```python
from build123d import *

# Parameters (mm, degrees)
BODY_SKETCH_W       = 31.8
BODY_SKETCH_H       = 20.9
BODY_DEPTH          = 9.9
NUT_X_SKETCH_W      = 16.85
NUT_X_SKETCH_H      = 9.45
NUT_X_SKETCH_2_W    = 16.85
NUT_X_SKETCH_2_H    = 9.45
SOCKET_X_SKETCH_W   = 17.8
SOCKET_X_SKETCH_H   = 4.7625
SOCKET_X_SKETCH_2_W = 17.8
SOCKET_X_SKETCH_2_H = 4.7625


with BuildPart() as part:
    # Body Sketch → Body (new, symmetric)
    with BuildSketch(Plane.XY):
        with Locations((0, 0.75)):
            Rectangle(BODY_SKETCH_W, BODY_SKETCH_H)
    extrude(amount=BODY_DEPTH, both=True)

    # Nut _X Sketch → Nut _X (revolve)
    with BuildSketch(Plane.XY, mode=Mode.PRIVATE) as nut_x_sk:
        with Locations((24.325, 4.725)):
            Rectangle(NUT_X_SKETCH_W, NUT_X_SKETCH_H)
    revolve(nut_x_sk.sketch.rotate(Axis((-1000, 0, 0), (1, 0, 0)), 90), axis=Axis((-1000, 0, 0), (1, 0, 0)))

    # Nut -X Sketch 2 → Nut -X 2 (revolve)
    with BuildSketch(Plane.XY, mode=Mode.PRIVATE) as nut_x_2_sk:
        with Locations((-24.325, 4.725)):
            Rectangle(NUT_X_SKETCH_2_W, NUT_X_SKETCH_2_H)
    revolve(nut_x_2_sk.sketch.rotate(Axis((-1000, 0, 0), (1, 0, 0)), 90), axis=Axis((-1000, 0, 0), (1, 0, 0)))

    # Socket _X Sketch → Socket _X (revolve, cut)
    with BuildSketch(Plane.XY, mode=Mode.PRIVATE) as socket_x_sk:
        with Locations((24.85, 2.38125)):
            Rectangle(SOCKET_X_SKETCH_W, SOCKET_X_SKETCH_H)
    revolve(socket_x_sk.sketch.rotate(Axis((-1000, 0, 0), (1, 0, 0)), 90), axis=Axis((-1000, 0, 0), (1, 0, 0)), mode=Mode.SUBTRACT)

    # Socket -X Sketch 2 → Socket -X 2 (revolve, cut)
    with BuildSketch(Plane.XY, mode=Mode.PRIVATE) as socket_x_2_sk:
        with Locations((-24.85, 2.38125)):
            Rectangle(SOCKET_X_SKETCH_2_W, SOCKET_X_SKETCH_2_H)
    revolve(socket_x_2_sk.sketch.rotate(Axis((-1000, 0, 0), (1, 0, 0)), 90), axis=Axis((-1000, 0, 0), (1, 0, 0)), mode=Mode.SUBTRACT)

    # Stem Sketch → Stem (revolve)
    with BuildSketch(Plane.XY, mode=Mode.PRIVATE) as stem_sk:
        Polygon((0, 11.2), (9.85, 11.2), (9.85, 15.4), (14, 15.4), (14, 19.9), (9.85, 19.9), (9.85, 21.5), (3, 21.5), (3, 31), (0, 31), align=None)
    revolve(stem_sk.sketch.rotate(Axis((0, -500, 0), (0, 1, 0)), 90), axis=Axis((0, -500, 0), (0, 1, 0)))


solid = part.part
```
Geometry: final body of the model. Coordinates: model frame, mm. A direction names the side the tool comes from. Coordinates: 2 decimals unless noted, no trailing zeros. Order: outer loops, then holes, each group sorted by start corner. A loop starts at its lowest first (then second) coordinate and runs counter-clockwise, first axis right, second up. Notation, with made-up numbers: (-35, -8.5) - (-21, -8.5) arc R20 cw to (-21, -0.5) - close; hole circle Ø1 at (-25, -37). An arc over 180 degrees is marked (long way). Return JSON: item names as keys, results as strings. Group by question number.
1. Cut plane A-A (y = 0). Output: boundary loops of the cut face in (x, z).
2. Pull-direction query (Y, two-part tool) for faces 1 (the face through (15.9, 9, 4)), 2 (the face through (24.47, 4.65, -1.03)), 3 (the face through (24.443, -2.839, 9.014)), 4 (the face through (-10, 19.9, -3)); classes: pulls with the +Y half, pulls with the -Y half, needs draft (parallel to the pull), parting line crosses it, or undercut.
3. Set-up query: faces 5 (the face through (0, 1, 9.9)), 6 (the face through (-10, 15.4, 3)), 7 (the face through (12.4, 17.7, -6.5)), 8 (the face through (-24.23, 4.65, -1.03)). Return all of +Z, -Z, +X, -X, +Y, -Y with unobstructed straight access to the full face (end or side cutting, diameter ignored); none if empty.
4. Material intervals for line 1 along Y through (x, z) = (-2, 9.75); line 2 along Y through (x, z) = (-26.75, 0); line 3 along Z through (x, y) = (-7, 4), sorted ascending. Write a range as [from, to].
5. Pin query (flat end, axial travel): pin 1 (1.5 mm diameter, centred on x = -16, z = -3, fed in from -Y); pin 2 (6 mm diameter, centred on y = 11, z = -7.5, fed in from +X); pin 3 (3 mm diameter, centred on x = 3.5, y = -4.5, fed in from +Z); pin 4 (6 mm diameter, centred on x = 14, y = 18, fed in from +Z). Return the tip coordinate at first contact, or that it passes through.
6. Cut plane B-B (x = 0). Output: boundary loops of the cut face in (y, z).
7. Cut plane C-C (z = 6.75). Output: boundary loops of the cut face in (x, y).
Resolved:
{
 "1": {"outline": "(-32.75, -9.45) - (-15.9, -9.45) - (-15.9, -9.9) - (15.9, -9.9) - (15.9, -9.45) - (32.75, -9.45) - (32.75, -4.76) - (15.95, -4.76) - (15.95, 4.76) - (32.75, 4.76) - (32.75, 9.45) - (15.9, 9.45) - (15.9, 9.9) - (-15.9, 9.9) - (-15.9, 9.45) - (-32.75, 9.45) - (-32.75, 4.76) - (-15.95, 4.76) - (-15.95, -4.76) - (-32.75, -4.76) - close"},
 "2": {"face 1": "needs draft", "face 2": "undercut", "face 3": "parting line crosses it", "face 4": "pulls with the +Y half"},
 "3": {"face 5": "+Z, +X, -X, -Y", "face 6": "none", "face 7": "+Y", "face 8": "-X"},
 "4": {"line 1": "y = [-9.7, 11.2], [15.4, 19.9]", "line 2": "y = [-9.45, -4.76], [4.76, 9.45]", "line 3": "z = [-9.9, 9.9]"},
 "5": {"pin 1": "stops at y = -9.7", "pin 2": "stops at x = 15.9", "pin 3": "stops at z = 9.9", "pin 4": "stops at z = 8.66"},
 "6": {"outline": "(-9.7, -9.9) - (11.2, -9.9) - (11.2, -9.85) - (15.4, -9.85) - (15.4, -14) - (19.9, -14) - (19.9, -9.85) - (21.5, -9.85) - (21.5, -3) - (31, -3) - (31, 3) - (21.5, 3) - (21.5, 9.85) - (19.9, 9.85) - (19.9, 14) - (15.4, 14) - (15.4, 9.85) - (11.2, 9.85) - (11.2, 9.9) - (-9.7, 9.9) - close"},
 "7": {"outline": "(-32.75, -6.61) - (-15.9, -6.61) - (-15.9, -9.7) - (15.9, -9.7) - (15.9, -6.61) - (32.75, -6.61) - (32.75, 6.61) - (15.9, 6.61) - (15.9, 11.2) - (7.17, 11.2) - (7.17, 15.4) - (12.27, 15.4) - (12.27, 19.9) - (7.17, 19.9) - (7.17, 21.5) - (-7.17, 21.5) - (-7.17, 19.9) - (-12.27, 19.9) - (-12.27, 15.4) - (-7.17, 15.4) - (-7.17, 11.2) - (-15.9, 11.2) - (-15.9, 6.61) - (-32.75, 6.61) - close"}
}
